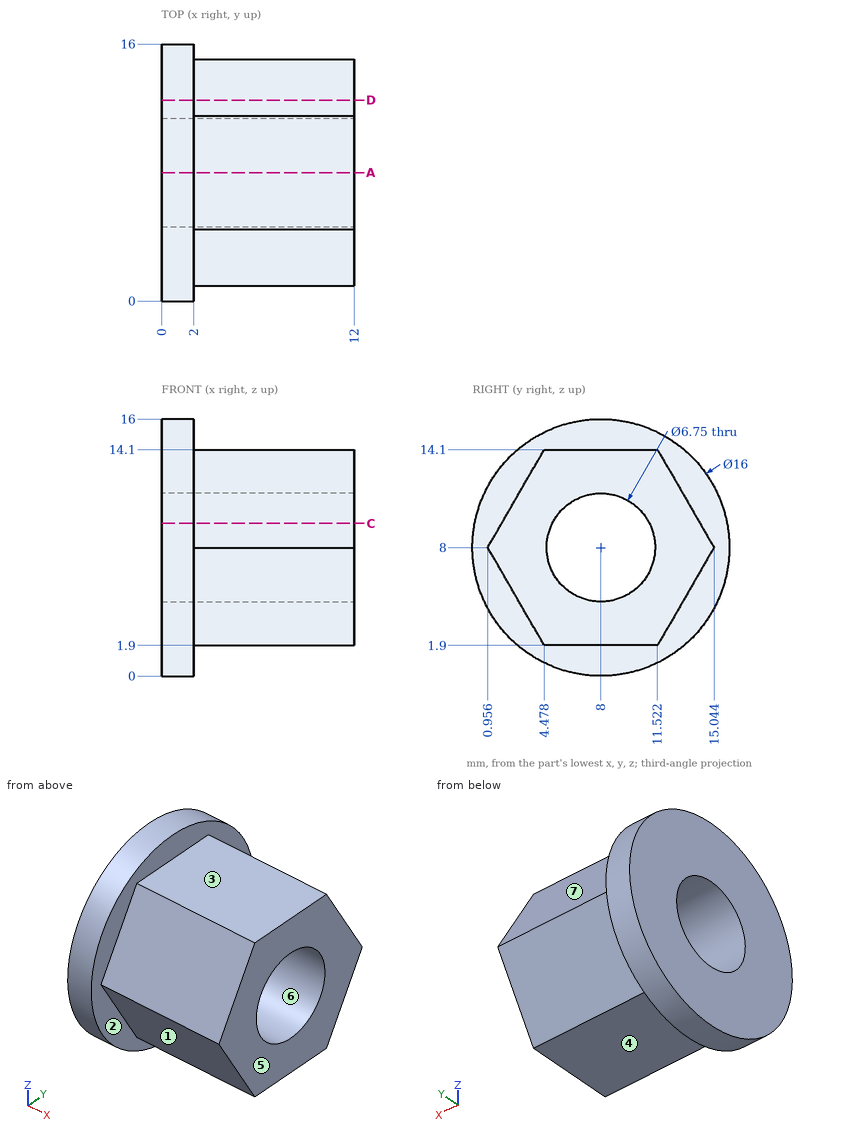
Check sheet for the drawn part. Datum: minimum x, y, z corner. Units: mm. A direction names the side the tool comes from. Coordinates: 2 decimals unless noted, no trailing zeros. Loops run counter-clockwise (first coordinate to the right, second up) from the corner with the lowest first, then second, coordinate; pieces in that order, holes last. Notation, with made-up numbers: (-30, 13) -> (-22, 13) arc R10 ccw to (-22, 28) -> close; hole circle Ø11 at (-13, 79). An arc over 180 degrees is marked (long way). Answer in a Markdown table with one row per item.
1. Sectioned sample at C-C, the plane z = 9.5. Record the boundary of the cut face in (x, y).
Check values:
| item | result |
|---|---|
| outline | (0, 0.14) -> (2, 0.14) -> (2, 1.82) -> (12, 1.82) -> (12, 4.98) -> (0, 4.98) -> close; (0, 11.02) -> (12, 11.02) -> (12, 14.18) -> (2, 14.18) -> (2, 15.86) -> (0, 15.86) -> close |
2. Access from +Z, -Z, +X, -X, +Y, -Y to the whole of each face (thin tool, end or side, straight path). Record for the marked faces 1, 2 and 3.
Check values:
| item | result |
|---|---|
| face 1 | -Z, +X, -Y |
| face 2 | +X |
| face 3 | +Z, +X, +Y, -Y |
3. Release check for a two-part mould opening along Z. For the marked faces 4, 5, 6 and 7 record: released by +Z, released by -Z, zero draft, split by the parting line, or undercut.
Check values:
| item | result |
|---|---|
| face 4 | released by -Z |
| face 5 | zero draft |
| face 6 | undercut |
| face 7 | released by +Z |
4. Go/stop test with flat-tipped pins: pin 1 (5.5 mm diameter, centred on x = 8.5, y = 9, fed in from +Z); pin 2 (5.5 mm diameter, centred on x = 8, y = 7, fed in from -Z); pin 3 (4 mm diameter, centred on x = 3.5, z = 3, fed in from +Y) (1 decimal). Record where each tip stops, or that it passes through.
Check values:
| item | result |
|---|---|
| pin 1 | stops at z = 14.1 |
| pin 2 | stops at z = 1.9 |
| pin 3 | stops at y = 15.1 |
5. Material ranges on line 1 along X through (y, z) = (7.25, 1.75); line 2 along Z through (x, y) = (10.5, 9.5); line 3 along Y through (x, z) = (8, 6.75) (1 decimal), recorded low to high. Write a range as [from, to].
Check values:
| item | result |
|---|---|
| line 1 | x = [0, 2] |
| line 2 | z = [1.9, 4.98], [11.02, 14.1] |
| line 3 | y = [1.7, 4.9], [11.1, 14.3] |
6. Sectioned sample at A-A, the plane y = 8. Record the boundary of the cut face in (x, z) (1 decimal).
Check values:
| item | result |
|---|---|
| outline | (0, 0) -> (2, 0) -> (2, 1.9) -> (12, 1.9) -> (12, 4.6) -> (0, 4.6) -> close; (0, 11.4) -> (12, 11.4) -> (12, 14.1) -> (2, 14.1) -> (2, 16) -> (0, 16) -> close |
7. Sectioned sample at D-D, the plane y = 12.5. Record the boundary of the cut face in (x, z).
Check values:
| item | result |
|---|---|
| outline | (0, 1.39) -> (2, 1.39) -> (2, 3.59) -> (12, 3.59) -> (12, 12.41) -> (2, 12.41) -> (2, 14.61) -> (0, 14.61) -> close |
